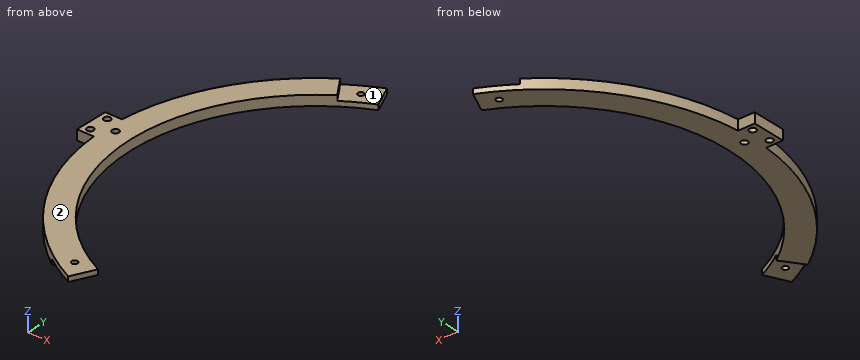
from build123d import *

# Parameters (mm, degrees)
ESQUISSE1_R             = 2
BOSS_EXTRU_1_DEPTH      = 6
ESQUISSE3_R             = 1.75
ENL_V_MAT_EXTRU_1_DEPTH = 10
ENL_V_START             = -3
ENL_V_MAT_EXTRU_2_DEPTH = 3
ENL_V_MAT_EXTRU_3_DEPTH = 3


with BuildPart() as part:
    # Esquisse1 → Boss.-Extru.1 (new body)
    with BuildSketch(Plane.XY):
        with BuildLine():
            Line((-134.599357944, -10), (-124.599357944, -10))
            ThreePointArc((-124.599357944, -10), (-102.650769054, -71.328953537), (-52.827282718, -113.28847338))
            Line((-52.827282718, -113.28847338), (-46.488008791, -99.693856574))
            ThreePointArc((-46.488008791, -99.693856574), (-110, 0), (-46.488008791, 99.693856574))
            Line((-46.488008791, 99.693856574), (-52.827282718, 113.28847338))
            ThreePointArc((-52.827282718, 113.28847338), (-102.650769054, 71.328953537), (-124.599357944, 10))
            Line((-124.599357944, 10), (-134.599357944, 10))
            Line((-134.599357944, 10), (-134.599357944, -10))
        make_face()
        with Locations((-120, 0)):
            Circle(ESQUISSE1_R, mode=Mode.SUBTRACT)
        with Locations((-130, 6)):
            Circle(ESQUISSE1_R, mode=Mode.SUBTRACT)
        with Locations((-130, -6)):
            Circle(ESQUISSE1_R, mode=Mode.SUBTRACT)
    extrude(amount=BOSS_EXTRU_1_DEPTH)

    # Esquisse3 → Enlèv. mat.-Extru.1 (cut)
    with BuildSketch(Plane.XY.offset(6)):
        with Locations((-58.75, 101.757984945)):
            Circle(ESQUISSE3_R)
        with Locations((-58.75, -101.757984945)):
            Circle(ESQUISSE3_R)
    extrude(amount=-ENL_V_MAT_EXTRU_1_DEPTH, mode=Mode.SUBTRACT)

    # Esquisse4 → Enlèv. mat.-Extru.2 (cut)
    with BuildSketch(Plane.XY.offset(6).offset(ENL_V_START)):
        with BuildLine():
            Line((-71.697054544, 102.394005536), (-63.093407999, 90.106724872))
            ThreePointArc((-63.093407999, 90.106724872), (-55, 95.262794416), (-46.488008791, 99.693856574))
            Line((-46.488008791, 99.693856574), (-52.827282718, 113.28847338))
            ThreePointArc((-52.827282718, 113.28847338), (-62.5, 108.253175473), (-71.697054544, 102.394005536))
        make_face()
    extrude(amount=ENL_V_MAT_EXTRU_2_DEPTH, mode=Mode.SUBTRACT)

    # Esquisse6 → Enlèv. mat.-Extru.3 (cut)
    with BuildSketch(Plane(origin=(0, 0, 0), x_dir=(-1, 0, 0), z_dir=(0, 0, -1))):
        with BuildLine():
            Line((63.093407999, -90.106724872), (71.697054544, -102.394005536))
            ThreePointArc((71.697054544, -102.394005536), (62.5, -108.253175473), (52.827282718, -113.28847338))
            Line((52.827282718, -113.28847338), (46.488008791, -99.693856574))
            ThreePointArc((46.488008791, -99.693856574), (55, -95.262794416), (63.093407999, -90.106724872))
        make_face()
    extrude(amount=-ENL_V_MAT_EXTRU_3_DEPTH, mode=Mode.SUBTRACT)


solid = part.part
Work out the finished part from the listing and answer in its coordinate system (mm). Face numbers are marked on the shaded views. A direction names the side the tool comes from. Give positions to 0.01 mm unless a question says otherwise; leave off trailing zeros. Loops run counter-clockwise (first coordinate to the right, second up) from the corner with the lowest first, then second, coordinate; pieces in that order, holes last. Notation, with made-up numbers: (-8.5, 65.5) -> (22.5, 65.5) arc R30 ccw to (22.5, 97.5) -> close; hole circle Ø1 at (6, 27). An arc over 180 degrees is marked (long way). Use a Markdown table: item, result. Add a question column.
1) The part is cut by section C-C, the plane x = -130. Determine the outline of the cut face in (y, z), plus the area to 3 significant figures.
2) The part is cut by section D-D, the plane z = 1.65. Determine the outline of the cut face in (x, y), plus the area to 3 significant figures.
3) Which of the six approach directions +Z, -Z, +X, -X, +Y, -Y give full straight-line access (tool end or side, diameter ignored) to the marked faces 1 and 2?
4) Each of these flat-tipped pins is pushed along its axis until it touches: P1, Ø3, axis at y = -5, z = 5, coming from the +X side; P2, Ø3, axis at x = -130, y = 6, coming from the +Z side; P3, Ø1.5, axis at x = -72.5, z = 4.5, coming from the -Y side; P4, Ø1.5, axis at x = -88.5, z = 5.5, coming from the +Y side. Where does it stop, or does it pass through?
5) Consider line 1 along Y through (x, z) = (-130, 2.5); line 2 along Y through (x, z) = (-126, 2.5); line 3 along Y through (x, z) = (-87.5, 1.3). Determine where each line is inside the solid, lowest interval first.
6) The part is cut by section A-A, the plane y = 0. Determine the outline of the cut face in (x, z), plus the area to 3 significant figures.
7) The part is cut by section B-B, the plane x = -120. Determine the outline of the cut face in (y, z), plus the area to 3 significant figures.
Reported:
| question | item | result |
|---|---|---|
| 1 | outline | (-10, 0) -> (-8, 0) -> (-8, 6) -> (-10, 6) -> close; (-4, 0) -> (4, 0) -> (4, 6) -> (-4, 6) -> close; (8, 0) -> (10, 0) -> (10, 6) -> (8, 6) -> close |
| 1 | area | 72.0 mm^2 |
| 2 | outline | (-134.6, -10) -> (-124.6, -10) arc R125 ccw to (-71.7, -102.39) -> (-63.09, -90.11) arc R110 cw to (-46.49, 99.69) -> (-52.83, 113.29) arc R125 ccw to (-124.6, 10) -> (-134.6, 10) -> close; hole circle Ø4 at (-130, -6); hole circle Ø4 at (-130, 6); hole circle Ø4 at (-120, 0); hole circle Ø3.5 at (-58.75, 101.76) |
| 2 | area | 3,840 mm^2 |
| 3 | face 1 | +Z, +X, +Y |
| 3 | face 2 | +Z, +X, -X, +Y, -Y |
| 4 | P1 | stops at x = -109.81 |
| 4 | P2 | passes through |
| 4 | P3 | stops at y = -102.36 |
| 4 | P4 | stops at y = 89.02 |
| 5 | line 1 | y = -10 to -8, -4 to 4, 8 to 10 |
| 5 | line 2 | y = -10 to 10 |
| 5 | line 3 | y = -89.27 to -66.66, 66.66 to 89.27 |
| 6 | outline | (-134.6, 0) -> (-122, 0) -> (-122, 6) -> (-134.6, 6) -> close; (-118, 0) -> (-110, 0) -> (-110, 6) -> (-118, 6) -> close |
| 6 | area | 124 mm^2 |
| 7 | outline | (-35, 0) -> (-2, 0) -> (-2, 6) -> (-35, 6) -> close; (2, 0) -> (35, 0) -> (35, 6) -> (2, 6) -> close |
| 7 | area | 396 mm^2 |
